The model under review builds one solid part; all positions refer to its coordinate system, in mm. A direction names the side the tool comes from. Give positions to 0.01 mm unless a question says otherwise; leave off trailing zeros. Order: outer loops, then holes, each group sorted by start corner. A loop starts at its lowest first (then second) coordinate and runs counter-clockwise, first axis right, second up.
```python
from build123d import *

# Parameters (mm, degrees)
F1_DEPTH = 5.08
F2_T     = -2.54


with BuildPart() as f1:
    # F0 (on Front) → F1 (new body)
    with BuildSketch(Plane.XZ):
        with BuildLine():
            Line((-5.585341, -13.793164), (5.585341, -13.793164))
            ThreePointArc((5.585341, -13.793164), (8.279418, -12.677241), (9.395341, -9.983164))
            Line((9.395341, -9.983164), (9.395341, 9.983164))
            ThreePointArc((9.395341, 9.983164), (8.279418, 12.677241), (5.585341, 13.793164))
            Line((5.585341, 13.793164), (-5.585341, 13.793164))
            ThreePointArc((-5.585341, 13.793164), (-8.279418, 12.677241), (-9.395341, 9.983164))
            Line((-9.395341, 9.983164), (-9.395341, -9.983164))
            ThreePointArc((-9.395341, -9.983164), (-8.279418, -12.677241), (-5.585341, -13.793164))
        make_face()
    extrude(amount=F1_DEPTH)

    # F2
    f2_openings = [f1.faces().sort_by_distance(p)[0] for p in [
        (0, -5.08, 0),
    ]]
    offset(amount=F2_T, openings=f2_openings)


solid = f1.part
```
Item 1: Take a section at B-B (z = 2.5). Give the boundary of the cut face in (x, y), and give its area (3 significant figures).
Values found:
outline: (-9.4, -5.08) - (-6.86, -5.08) - (-6.86, -2.54) - (6.86, -2.54) - (6.86, -5.08) - (9.4, -5.08) - (9.4, 0) - (-9.4, 0) - close
area: 60.6 mm2
Item 2: Draft analysis for pull direction X (two halves, no side actions). For faces 1 (the flat face through (0, -4, 11.253)), 2 (the flat face through (0, 0, 0)), 3 (the cylindrical face through (-6.473, -3.792, 10.891)), 4 (the cylindrical face through (-8.25, -2.504, 12.707)), state which applies: released by +X, released by -X, zero draft, split by the parting line, or undercut.
Values found:
face 1: undercut
face 2: zero draft
face 3: undercut
face 4: released by -X
Item 3: For line 1 (Z direction, x = -4, y = -3.85); line 2 (X direction, y = -4.4, z = -2.75); line 3 (Z direction, x = 5.75, y = -3.9), list the stretches that pass through material, from the lowest coordinate up.
Values found:
line 1: z = -13.79 to -11.25, 11.25 to 13.79
line 2: x = -9.4 to -6.86, 6.86 to 9.4
line 3: z = -13.79 to -11.24, 11.24 to 13.79
Item 4: For faces 5 (the flat face through (0, -2.54, 0)), 6 (the flat face through (0, -3, -13.793)), list the 3-axis set-ups (+Z, -Z, +X, -X, +Y, -Y) from which the entire face can be reached by the end or side of a thin tool; tool diameter is ignored.
Values found:
face 5: -Y
face 6: -Z, +X, -X, +Y, -Y
Item 5: Take a section at C-C (y = -1.35). Give the boundary of the cut face in (x, z).
Values found:
outline: (-9.4, -9.98) arc R3.81 ccw to (-5.59, -13.79) - (5.59, -13.79) arc R3.81 ccw to (9.4, -9.98) - (9.4, 9.98) arc R3.81 ccw to (5.59, 13.79) - (-5.59, 13.79) arc R3.81 ccw to (-9.4, 9.98) - close
Item 6: Clearance check with a flat-ended pin moving along its axis: pin 1 Ø11 at (x, z) = (0.5, -4) entering from -Y. State where the tip first meets the part, or that it passes through.
Values found:
pin 1: stops at y = -2.54
Item 7: Take a section at A-A (y = -3.25). Give the boundary of the cut face in (x, z), and give its area (3 significant figures).
Values found:
outline: (-9.4, -9.98) arc R3.81 ccw to (-5.59, -13.79) - (5.59, -13.79) arc R3.81 ccw to (9.4, -9.98) - (9.4, 9.98) arc R3.81 ccw to (5.59, 13.79) - (-5.59, 13.79) arc R3.81 ccw to (-9.4, 9.98) - close; hole (-6.86, -9.98) arc R1.27 ccw to (-5.59, -11.25) - (5.59, -11.25) arc R1.27 ccw to (6.86, -9.98) - (6.86, 9.98) arc R1.27 ccw to (5.59, 11.25) - (-5.59, 11.25) arc R1.27 ccw to (-6.86, 9.98) - close
area: 199 mm2
